Verification items for the finished model (mm, model axes). Give positions to 0.01 mm unless a question says otherwise; leave off trailing zeros. Loops run counter-clockwise (first coordinate to the right, second up) from the corner with the lowest first, then second, coordinate; pieces in that order, holes last. Notation, with made-up numbers: M 18.5,-5 L 65.5,-5 A11 ccw 65.5,8 Z; hole C -32.75,71 d4. An arc over 180 degrees is marked long. Use a Markdown table: item, result.
Autodesk Inventor part; units mm, degrees
ref_plane "YZ Plane" through (0, 0, 0) normal (1, 0, 0) x (0, 1, 0)
ref_plane "XZ Plane" through (0, 0, 0) normal (0, 1, 0) x (-1, 0, 0)
ref_plane "XY Plane" through (0, 0, 0) normal (0, 0, 1) x (1, 0, 0)
sketch "Sketch1" plane through (0, 0, 0) normal (0, 0, 1) x (1, 0, 0)
  arc A0 (34.8698, 1.9636) -> (-30.2459, 17.4625) centre (0, 0) ccw
  line L0 (-30.2459, 17.4625) -> (-41.2445, 23.8125)
  line L1 (0, 0) -> (-58.2409, 0) construction
  line L2 (47.853, -228.6) -> (34.8698, 1.9636)
  line L3 (82.55, -393.7) -> (47.4407, 4.1861)
  line L4 (57.15, -393.7) -> (82.55, -393.7)
  circle A1 centre (69.155, -381) radius 3.175
  line L5 (47.5493, 47.625) -> (47.5493, 2.9548)
  line L6 (-41.2445, 47.625) -> (-41.2445, 23.8125)
  line L7 (-41.2445, 47.625) -> (161.9555, 47.625) construction
  line L8 (-41.2445, 47.625) -> (161.9555, 47.625) construction
  line L9 (-41.2445, 47.625) -> (161.9555, 47.625) construction
  line L10 (-41.2445, 47.625) -> (161.9555, 47.625) construction
  line L11 (-41.2445, 47.625) -> (47.5493, 47.625)
  line L12 (47.853, -228.6) -> (57.15, -393.7)
  circle A2 centre (59.69, -255.905) radius 2.3813
  circle A3 centre (34.8493, 34.925) radius 3.175
  point P0 (47.5493, 25.2899)
  point P1 (51.4288, -292.1)
  dimension "d0" = 69.85
  dimension "d1" = 30
  dimension "d2" = 57.15
  dimension "d3" = 25.4
  dimension "d4" = 393.7
  dimension "d5" = 6.35
  dimension "d6" = 12.7
  dimension "d7" = 12.7
  dimension "d72" = 4.7625
  dimension "d73" = 2.54
  dimension "d74" = 137.795
  dimension "d76" = 6.35
  dimension "d77" = 12.7
  dimension "d78" = 12.7
extrude "Plate10" add sketch "Sketch1" along normal blind 3.175
equation "\"BendRadius\" = Thickness"
equation "\"BendReliefWidth\" = Thickness"
equation "\"BendReliefDepth\" = 0.5 * Thickness"
equation "\"CornerReliefSize\" = 4 * Thickness"
equation "\"MinimumRemnant\" = 2 * Thickness"
equation "\"TransitionRadius\" = BendRadius"
equation "\"JacobiRadiusSize\" = BendRadius"
equation "\"GapSize\" = Thickness"
equation "\"d10\" = BendRadius"
equation "\"d28\" = BendRadius"
equation "\"d71\" = BendRadius"
equation "\"d75\" = BendRadius"
equation "\"d79\" = BendRadius"
properties part number "PassiveHooks2"
(1) Cross-section at A-A on z = 0.9. State how many separate pieces and enclosed holes the cut face has, then the cut area to 3 significant figures.
Results below:
| item | result |
|---|---|
| separate pieces | 1 |
| enclosed holes | 3 |
| area | 9,590 mm^2 |
(2) Draft check along X on faces 1 (the cylindrical face through (7.476, 34.115, 1.565)), 2 (the flat face through (65.295, -198.149, 1.565)), 3 (the flat face through (57, -156, 3.175)). Enter one of: +X half, -X half, draft (parallel to the pull), parting line (faces both ways), or undercut.
Results below:
| item | result |
|---|---|
| face 1 | undercut |
| face 2 | +X half |
| face 3 | draft |
(3) Material ranges on line 1 (X direction, y = -381, z = 2.05); line 2 (X direction, y = 1.5, z = 1.8); line 3 (X direction, y = -291.5, z = 1.2), recorded low to high.
Results below:
| item | result |
|---|---|
| line 1 | 56.43 to 65.98, 72.33 to 81.43 |
| line 2 | 34.9 to 47.68 |
| line 3 | 51.39 to 73.53 |
(4) Cross-section at B-B on y = -21.5. Record the cut outline in (x, z) (3 decimals), then the cut area to 3 significant figures.
Results below:
| item | result |
|---|---|
| outline | M 36.191,0 L 49.707,0 L 49.707,3.175 L 36.191,3.175 Z |
| area | 42.9 mm^2 |
(5) Cross-section at C-C on x = -26.5. Record the cut outline in (y, z) (3 decimals), then the cut area to 3 significant figures.
Results below:
| item | result |
|---|---|
| outline | M 22.749,0 L 47.625,0 L 47.625,3.175 L 22.749,3.175 Z |
| area | 79.0 mm^2 |
(6) Gauge pin test, flat end, axial feed: P1, Ø10, axis at x = 53.5, y = -51, coming from the +Z side (3 decimals). Record the tip position at first contact, or that the pin passes through.
Results below:
| item | result |
|---|---|
| P1 | z = 3.175 |
